```python
from build123d import *

# Parameters (mm, degrees)
SKETCH2_R             = 8
SKETCH2_R_2           = 3.75
BOSS_EXTRUDE1_DEPTH   = 20
BOSS_EXTRUDE1_2_DEPTH = 20
SKETCH4_W             = 164
SKETCH4_H             = 16
BOSS_EXTRUDE2_DEPTH   = 12
BOSS_EXTRUDE3_DEPTH   = 16
LPATTERN2_COUNT       = 24
LPATTERN2_PITCH       = 6.1


with BuildPart() as part:
    # Sketch2 → Boss-Extrude1 (new body)
    with BuildSketch(Plane(origin=(0, 0, 0), x_dir=(1, 0, 0), z_dir=(0, 1, 0))):
        with Locations(Location((-82, 0, 0), (0, 0, 270))):
            Circle(SKETCH2_R)
        with Locations(Location((-82, 0, 0), (0, 0, 270))):
            Circle(SKETCH2_R_2, mode=Mode.SUBTRACT)
    extrude(amount=BOSS_EXTRUDE1_DEPTH)



with BuildPart() as body_2:
    # Sketch2 → Boss-Extrude1 2 (new body)
    with BuildSketch(Plane(origin=(0, 0, 0), x_dir=(1, 0, 0), z_dir=(0, 1, 0))):
        with Locations(Location((82, 0, 0), (0, 0, 270))):
            Circle(SKETCH2_R)
        with Locations(Location((82, 0, 0), (0, 0, 270))):
            Circle(SKETCH2_R_2, mode=Mode.SUBTRACT)
    extrude(amount=BOSS_EXTRUDE1_2_DEPTH)


with BuildPart() as part_1:
    add(part.part)

    add(body_2.part)  # Boss-Extrude2 merges body 2
    # Sketch4 → Boss-Extrude2 (add)
    with BuildSketch(Plane(origin=(0, 16, 0), x_dir=(1, 0, 0), z_dir=(0, 1, 0))):
        Rectangle(SKETCH4_W, SKETCH4_H)
    extrude(amount=-BOSS_EXTRUDE2_DEPTH)

    # Sketch5 → Boss-Extrude3 (add, through all)
    with BuildSketch(Plane.XY.offset(8)):
        Polygon((72.909925586, 16), (72, 18.5), (70, 18.5), (69.090074414, 16), align=None)
    boss_extrude3 = extrude(amount=-BOSS_EXTRUDE3_DEPTH)

    # LPattern2: Boss-Extrude3 ×24
    with Locations(*[(-i * LPATTERN2_PITCH, 0, 0) for i in range(1, LPATTERN2_COUNT)]):
        add(boss_extrude3)


solid = part_1.part
```
Geometry check sheet. Reference: the model listing, model coordinates, mm. A direction names the side the tool comes from. Round coordinates to 2 decimals unless told otherwise and drop trailing zeros. Loops run counter-clockwise (first coordinate to the right, second up) from the corner with the lowest first, then second, coordinate; pieces in that order, holes last. Notation, with made-up numbers: (44, 71.5) - (59, 71.5) arc R20 ccw to (59, 80.5) - close; hole circle Ø4 at (43, -1). An arc over 180 degrees is marked (long way). Write item = value, one per line. Start each with the question number.
1. Depth check by flat-ended pin: pin 1 (0.6 mm diameter, centred on x = -50.5, z = 0.5, fed in from +Y); pin 2 (1.1 mm diameter, centred on x = 25, z = 2, fed in from +Y); pin 3 (5 mm diameter, centred on x = 69.5, z = 2, fed in from -Y). Enter the tip coordinate at first touch or a pass-through.
2. Thickness scan on line 1 (X direction, y = 11, z = 0); line 2 (X direction, y = 7, z = -3.25); line 3 (Y direction, x = 52, z = 3.5). Record the ranges inside material, lowest first.
3. Section check B-B on z = 0. Give the number of separate pieces and of enclosed holes in the cut face, then the cut area to 3 significant figures.
4. Mould release check, pull along X, two halves, no side actions. Record for faces 5 (the face through (-85.44, 20, -1.89)), 6 (the face through (-85.66, 9.86, -0.81)): released by +X, released by -X, zero draft, split by the parting line, or undercut.
5. Set-up check for faces 1 (the face through (-81, 16, 0)), 2 (the face through (85.718, 9.86, -0.488)), 3 (the face through (-81, 4, 0)), 4 (the face through (-82, 10, 0)): record each of +Z, -Z, +X, -X, +Y, -Y from which the full face is reachable in a straight line by a thin tool's end or side.
6. Section check A-A on y = 11.5. Enter the section's corners in (x, z), then the cut area to 3 significant figures.
Working result:
q1.pin_1 = 18.5
q1.pin_2 = 16
q1.pin_3 = 4
q2.line_1 = -90 to -85.75, -82 to 82, 85.75 to 90
q2.line_2 = -89.31 to -83.87, -82 to 82, 83.87 to 89.31
q2.line_3 = 4 to 18.5
q3.separate_pieces = 3
q3.enclosed_holes = 0
q3.area = 2,380 mm^2
q4.face_5 = zero draft
q4.face_6 = undercut
q5.face_1 = +Y
q5.face_2 = none
q5.face_3 = -Y
q5.face_4 = +Y, -Y
q6.outline = (-82, -8) - (82, -8) arc R8 ccw to (82, 8) - (-82, 8) arc R8 ccw to start; hole (-82, -3.75) - (-82, 3.75) arc R3.75 ccw to start; hole (82, -3.75) arc R3.75 ccw to (82, 3.75) - close
q6.area = 2,780 mm^2
